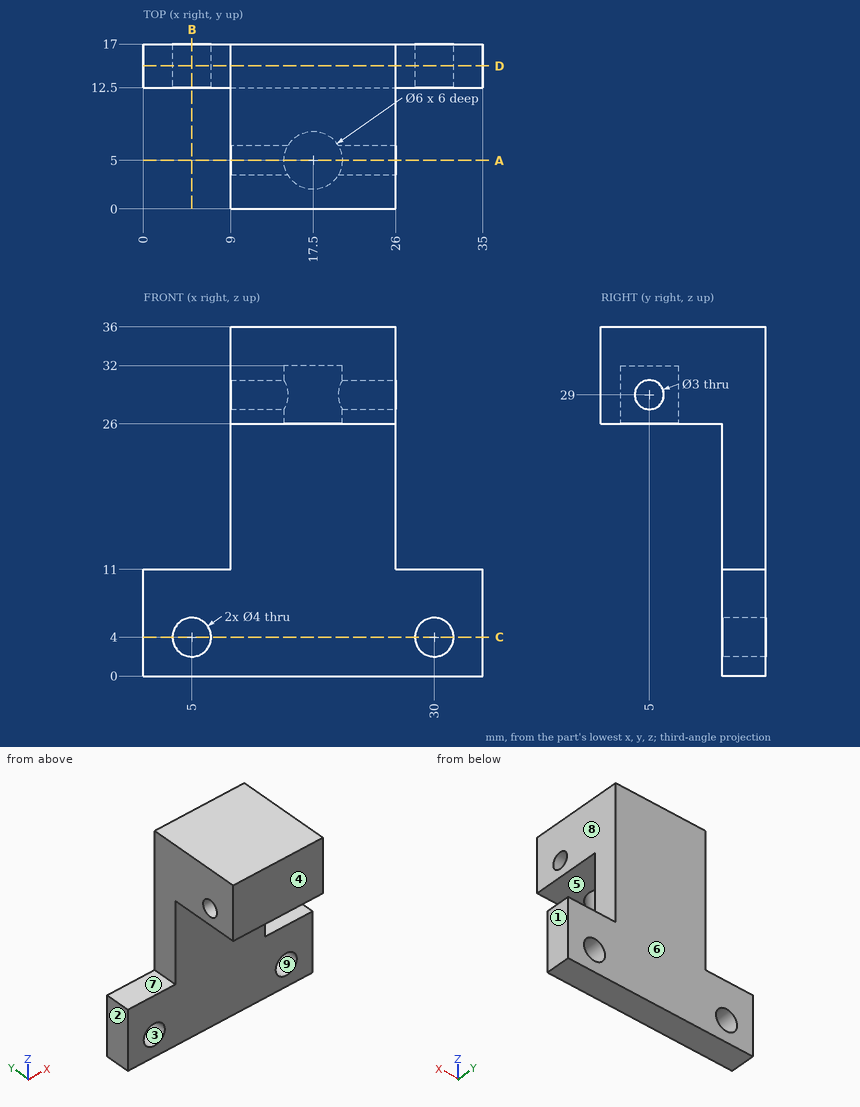
Could you check a few things on this drawing? It's one solid part, dimensions in mm from its lowest x, y, z. A direction names the side the tool comes from. Coordinates: 2 decimals unless noted, no trailing zeros. Order: outer loops, then holes, each group sorted by start corner. A loop starts at its lowest first (then second) coordinate and runs counter-clockwise, first axis right, second up.
1) Which directions (+Z, -Z, +X, -X, +Y, -Y) give clear straight access to the entire face, cutting with the end or side of a thin tool? Please do the marked faces 5, 6, 7, 8 and 9.
2) Imagine slicing it at A-A on y = 5. List the corners of the cut face in (x, z) for me.
3) Imagine slicing it at B-B on x = 5. List the corners of the cut face in (y, z) for me, and give its area (3 significant figures).
4) Will these pins go through, and if not, where does the flat tip stop? pin 1 (5 mm diameter, centred on y = 5, z = 29, fed in from -X); pin 2 (4 mm diameter, centred on y = 15, z = 28, fed in from +X); pin 3 (5 mm diameter, centred on x = 6, y = 15.5, fed in from +Z); pin 4 (3 mm diameter, centred on x = 5, z = 4, fed in from -Y).
5) We'd pull the mould along X, two halves only. Please class the marked faces 1, 2, 3 and 4: +X half, -X half, draft (parallel to the pull), parting line (faces both ways), or undercut.
6) Imagine slicing it at C-C on z = 4. List the corners of the cut face in (x, y) for me.
7) I need wall thicknesses on line 1 (Y direction, x = 17.5, z = 27.75); line 2 (X direction, y = 3.5, z = 28.5); line 3 (Z direction, x = 5, y = 16). Which ranges of each line are inside material? Lowest first, please.
8) Imagine slicing it at D-D on y = 14.75. List the corners of the cut face in (x, z) for me, and give its area (3 significant figures).
Response values:
1. face 5: -Z, +X, -X, -Y
1. face 6: +Z, -Z, +X, -X, +Y
1. face 7: +Z, -X, +Y, -Y
1. face 8: +Z, +X, +Y, -Y
1. face 9: +Y, -Y
2. outline: (9, 26) - (14.5, 26) - (14.5, 27.5) - (9, 27.5) - close; (9, 30.5) - (14.5, 30.5) - (14.5, 32) - (20.5, 32) - (20.5, 30.5) - (26, 30.5) - (26, 36) - (9, 36) - close; (20.5, 26) - (26, 26) - (26, 27.5) - (20.5, 27.5) - close
3. outline: (12.5, 0) - (17, 0) - (17, 2) - (12.5, 2) - close; (12.5, 6) - (17, 6) - (17, 11) - (12.5, 11) - close
3. area: 31.5 mm2
4. pin 1: stops at x = 9
4. pin 2: stops at x = 26
4. pin 3: stops at z = 11
4. pin 4: passes through
5. face 1: +X half
5. face 2: -X half
5. face 3: undercut
5. face 4: draft
6. outline: (0, 12.5) - (3, 12.5) - (3, 17) - (0, 17) - close; (7, 12.5) - (28, 12.5) - (28, 17) - (7, 17) - close; (32, 12.5) - (35, 12.5) - (35, 17) - (32, 17) - close
7. line 1: y = 0 to 2, 8 to 17
7. line 2: x = 9 to 14.9, 20.1 to 26
7. line 3: z = 0 to 2, 6 to 11
8. outline: (0, 0) - (35, 0) - (35, 11) - (26, 11) - (26, 36) - (9, 36) - (9, 11) - (0, 11) - close; hole circle Ø4 at (5, 4); hole circle Ø4 at (30, 4)
8. area: 785 mm2
